Part model, mm, in its own coordinate system. A direction names the side the tool comes from. Coordinates: 2 decimals unless noted, no trailing zeros. Order: outer loops, then holes, each group sorted by start corner. A loop starts at its lowest first (then second) coordinate and runs counter-clockwise, first axis right, second up. Notation, with made-up numbers: (4.25, -29) - (15.25, -29) arc R19 cw to (15.25, -20) - close; hole circle Ø6 at (53, 74.5). An arc over 180 degrees is marked (long way). Use a Markdown table: item, result. Add a question column.
1) Tool access for faces 1 (the face through (-15.64, 2.14, 45.75)), 2 (the face through (9.772, 0.493, -12.255)), 3 (the face through (-16.27, 0.54, 46.39)): list every direction of +Z, -Z, +X, -X, +Y, -Y with a clear straight run to the whole face (end or side of a thin tool).
2) Drop flat-ended pins along their axis: P1, Ø1.9, axis at x = -10.5, z = -10.5, coming from the -Y side; P2, Ø4, axis at x = -0.5, z = -1, coming from the +Y side; P3, Ø2.5, axis at x = 10.5, z = -10.5, coming from the +Y side; P4, Ø1, axis at y = 1.5, z = -39.5, coming from the +X side. Give the stop position or say it passes through.
3) Saw through at B-B on z = 0. List the corners of the cut face in (x, y) (3 decimals).
4) Wall check: L1, parallel to X at y = 2.7, z = 0 (3 decimals); L2, parallel to Z at x = -10.5, y = 0.2; L3, parallel to X at y = 0.4, z = -10.5. Give the ranges that are in metal, low to high. Write a range as [from, to].
5) Saw through at A-A on x = 0. List the corners of the cut face in (y, z) (3 decimals).
6) Two-plate mould, pull along X, no slides. Class faces 4 (the face through (-15.75, 2.14, -45.64)), 5 (the face through (-16.39, 0.54, -46.27)), 6 (the face through (-19, 5, -8)): +X half, -X half, draft (parallel to the pull), parting line (faces both ways), or undercut.
```python
from build123d import *

# Parameters (mm, degrees)
EXTRUDE_1_DEPTH              = 5
FILLET_1_R                   = 9
FILLET_2_R                   = 18
SHELL_1_T                    = -2
CHAMFER_1_SIZE               = 0.5
CHAMFER_2_SIZE               = 2
SKETCH_2_W                   = 27
SKETCH_2_H                   = 27
EXTRUDE_2_DEPTH              = 1
SKETCH_3_R                   = 3.975
EXTRUDE_3_DEPTH              = 1
FILLET_3_R                   = 3
HOLE_WIZARD_M2_1_D           = 2.1
HOLE_WIZARD_M2_1_CBORE_D     = 3.8
HOLE_WIZARD_M2_1_CBORE_DEPTH = 1
PATTERN_CIRCULAR_1_COUNT     = 4
SKETCH_6_R                   = 3.975
CUT_EXTRUDE_1_DEPTH          = 1
SKETCH_7_R                   = 2.5
CUT_EXTRUDE_2_DEPTH          = 2


with BuildPart() as part:
    # ｽｹｯﾁ1 → ﾎﾞｽ - 押し出し1 (new body)
    with BuildSketch(Plane(origin=(0, 0, 0), x_dir=(1, 0, 0), z_dir=(0, 1, 0))):
        with BuildLine():
            Line((-20, 50), (28.833147735, 50))
            ThreePointArc((28.833147735, 50), (44, 0), (28.833147735, -50))
            Line((28.833147735, -50), (-20, -50))
            Line((-20, -50), (-20, 50))
        make_face()
    extrude(amount=EXTRUDE_1_DEPTH)

    # ﾌｨﾚｯﾄ1
    fillet_1_edges = [part.edges().sort_by_distance(p)[0] for p in [
        (-20, 2.5, -50),
        (-20, 2.5, 50),
    ]]
    fillet(fillet_1_edges, radius=FILLET_1_R)

    # ﾌｨﾚｯﾄ2
    fillet_2_edges = [part.edges().sort_by_distance(p)[0] for p in [
        (28.833147735, 2.5, -50),
        (28.833147735, 2.5, 50),
    ]]
    fillet(fillet_2_edges, radius=FILLET_2_R)

    # ｼｪﾙ1
    shell_1_openings = [part.faces().sort_by_distance(p)[0] for p in [
        (9.782139289, 5, 0),
    ]]
    offset(amount=SHELL_1_T, openings=shell_1_openings, kind=Kind.INTERSECTION)

    # 面取り1
    chamfer_1_edges = [part.edges().sort_by_distance(p)[0] for p in [
        (-18, 2, 0),
        (3.749030993, 2, 48),
        (42, 2, 0),
        (3.749030993, 2, -48),
        (26.930802414, 2, -45.59738537),
        (26.930802414, 2, 45.59738537),
        (-15.949747468, 2, 45.949747468),
        (-15.949747468, 2, -45.949747468),
    ]]
    chamfer(chamfer_1_edges, length=CHAMFER_1_SIZE)

    # 面取り2
    chamfer_2_edges = [part.edges().sort_by_distance(p)[0] for p in [
        (-20, 0, 0),
        (3.749030993, 0, 50),
        (-17.363961031, 0, 47.363961031),
        (-17.363961031, 0, -47.363961031),
        (3.749030993, 0, -50),
        (44, 0, 0),
        (27.984894967, 0, 47.297058541),
        (27.984894967, 0, -47.297058541),
    ]]
    chamfer(chamfer_2_edges, length=CHAMFER_2_SIZE)

    # ｽｹｯﾁ2 → ﾎﾞｽ - 押し出し2 (add)
    with BuildSketch(Plane(origin=(0, 2, 0), x_dir=(1, 0, 0), z_dir=(0, 1, 0))):
        Rectangle(SKETCH_2_W, SKETCH_2_H)
    extrude(amount=EXTRUDE_2_DEPTH)

    # ｽｹｯﾁ3 → ﾎﾞｽ - 押し出し3 (add)
    with BuildSketch(Plane(origin=(0, 3, 0), x_dir=(1, 0, 0), z_dir=(0, 1, 0))):
        with Locations(Location((0, 0, 0), (0, 0, 270))):
            Circle(SKETCH_3_R)
    extrude(amount=EXTRUDE_3_DEPTH)

    # ﾌｨﾚｯﾄ3
    fillet_3_edges = [part.edges().sort_by_distance(p)[0] for p in [
        (13.5, 2.5, 13.5),
        (13.5, 2.5, -13.5),
        (-13.5, 2.5, -13.5),
        (-13.5, 2.5, 13.5),
    ]]
    fillet(fillet_3_edges, radius=FILLET_3_R)

    # M2 なべ頭ねじ用座ぐり穴1 (through all)
    with Locations(Plane(origin=(0, 0, 0), x_dir=(-1, 0, 0), z_dir=(0, -1, 0))):
        with Locations((10.5, 10.5)):
            hole_wizard_m2_1 = CounterBoreHole(HOLE_WIZARD_M2_1_D / 2, HOLE_WIZARD_M2_1_CBORE_D / 2, HOLE_WIZARD_M2_1_CBORE_DEPTH)

    # 円形ﾊﾟﾀｰﾝ1: M2 なべ頭ねじ用座ぐり穴1 ×4 about axis
    pattern_circular_1_axis = Axis((0, 0, 0), (0, 1, 0))
    for i in range(1, PATTERN_CIRCULAR_1_COUNT):
        add(hole_wizard_m2_1.rotate(pattern_circular_1_axis, i * 360 / PATTERN_CIRCULAR_1_COUNT), mode=Mode.SUBTRACT)

    # ｽｹｯﾁ6 → ｶｯﾄ - 押し出し1 (cut)
    with BuildSketch(Plane(origin=(0, 3, 0), x_dir=(1, 0, 0), z_dir=(0, 1, 0))):
        with BuildLine():
            Line((-7.994506037, -12.15), (7.994506037, -12.15))
            ThreePointArc((7.994506037, -12.15), (8.378679656, -8.378679656), (12.15, -7.994506037))
            Line((12.15, -7.994506037), (12.15, 7.994506037))
            ThreePointArc((12.15, 7.994506037), (8.378679656, 8.378679656), (7.994506037, 12.15))
            Line((7.994506037, 12.15), (-7.994506037, 12.15))
            ThreePointArc((-7.994506037, 12.15), (-7.62628447, 11.36125435), (-7.5, 10.5))
            ThreePointArc((-7.5, 10.5), (-9.076975053, 7.858977471), (-12.15, 7.994506037))
            Line((-12.15, 7.994506037), (-12.15, -7.994506037))
            ThreePointArc((-12.15, -7.994506037), (-9.076975053, -7.858977471), (-7.5, -10.5))
            ThreePointArc((-7.5, -10.5), (-7.62628447, -11.36125435), (-7.994506037, -12.15))
        make_face()
        with Locations(Location((0, 0, 0), (0, 0, 270))):
            Circle(SKETCH_6_R, mode=Mode.SUBTRACT)
    extrude(amount=-CUT_EXTRUDE_1_DEPTH, mode=Mode.SUBTRACT)

    # ｽｹｯﾁ7 → ｶｯﾄ - 押し出し2 (cut)
    with BuildSketch(Plane(origin=(0, 4, 0), x_dir=(1, 0, 0), z_dir=(0, 1, 0))):
        with Locations(Location((0, 0, 0), (0, 0, 270))):
            Circle(SKETCH_7_R)
    extrude(amount=-CUT_EXTRUDE_2_DEPTH, mode=Mode.SUBTRACT)


solid = part.part
```
Results are:
| question | item | result |
|---|---|---|
| 1 | face 1 | +Y |
| 1 | face 2 | -Y |
| 1 | face 3 | +Z, -X, -Y |
| 2 | P1 | through |
| 2 | P2 | y = 4 |
| 2 | P3 | y = 3 |
| 2 | P4 | x = 34.92 |
| 3 | outline | (-20, 2) - (-18, 0) - (42, 0) - (44, 2) - (44, 5) - (42, 5) - (42, 2.5) - (41.5, 2) - (13.5, 2) - (13.5, 3) - (12.15, 3) - (12.15, 2) - (3.975, 2) - (3.975, 4) - (2.5, 4) - (2.5, 2) - (-2.5, 2) - (-2.5, 4) - (-3.975, 4) - (-3.975, 2) - (-12.15, 2) - (-12.15, 3) - (-13.5, 3) - (-13.5, 2) - (-17.5, 2) - (-18, 2.5) - (-18, 5) - (-20, 5) - close |
| 4 | L1 | [-20, -18], [-13.5, -12.15], [-3.975, -2.5], [2.5, 3.975], [12.15, 13.5], [42, 44] |
| 4 | L2 | [-48.2, -12.4], [-8.6, 8.6], [12.4, 48.2] |
| 4 | L3 | [-18.4, -12.4], [-8.6, 8.6], [12.4, 41.77] |
| 5 | outline | (0, -48) - (2, -50) - (5, -50) - (5, -48) - (2.5, -48) - (2, -47.5) - (2, -13.5) - (3, -13.5) - (3, -12.15) - (2, -12.15) - (2, -3.975) - (4, -3.975) - (4, -2.5) - (2, -2.5) - (2, 2.5) - (4, 2.5) - (4, 3.975) - (2, 3.975) - (2, 12.15) - (3, 12.15) - (3, 13.5) - (2, 13.5) - (2, 47.5) - (2.5, 48) - (5, 48) - (5, 50) - (2, 50) - (0, 48) - close |
| 6 | face 4 | undercut |
| 6 | face 5 | -X half |
| 6 | face 6 | draft |
